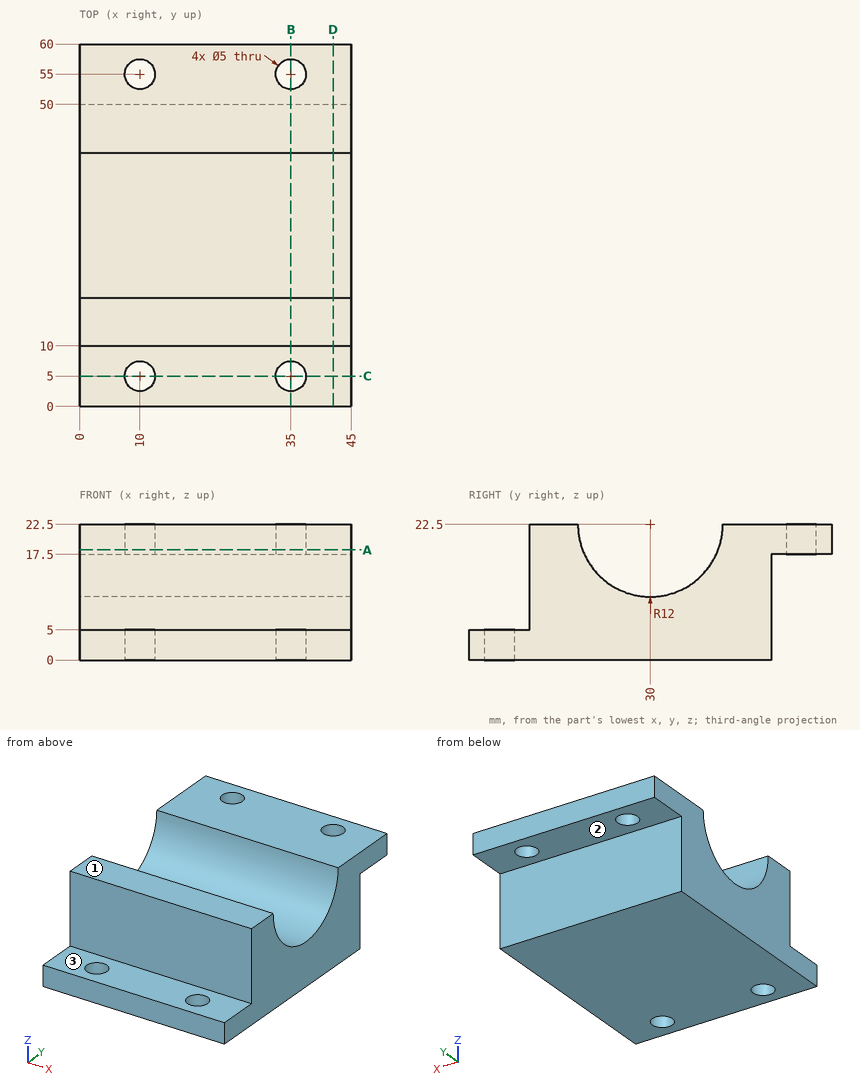
Can you work these out from the drawing? Everything is in mm from the part's minimum corner. A direction names the side the tool comes from. Give positions to 0.01 mm unless a question says otherwise; leave off trailing zeros. Loops run counter-clockwise (first coordinate to the right, second up) from the corner with the lowest first, then second, coordinate; pieces in that order, holes last. Notation, with made-up numbers: (49.5, -12) - (78.5, -12) arc R20 cw to (78.5, 12) - close; hole circle Ø6 at (70, 59.25). An arc over 180 degrees is marked (long way). Use one line per item in the form item = value.
1. I want a section at A-A (z = 18.25). Please give me the cut outline in (x, y).
Response values:
outline = (0, 10) - (45, 10) - (45, 18.78) - (0, 18.78) - close; (0, 41.22) - (45, 41.22) - (45, 60) - (0, 60) - close; hole circle Ø5 at (10, 55); hole circle Ø5 at (35, 55)
2. I'm going to push flat-ended pins straight in: pin 1 Ø4 at (x, z) = (34, 5.5) entering from +Y; pin 2 Ø8 at (x, y) = (35, 5) entering from -Z; pin 3 Ø8 at (x, y) = (31.5, 4) entering from +Z; pin 4 Ø8 at (x, y) = (10, 55) entering from -Z. Where does each tip first touch, or does it pass through?
Response values:
pin_1 = 50
pin_2 = 0
pin_3 = 5
pin_4 = 17.5
3. I want a section at D-D (x = 42). Please give me the cut outline in (y, z).
Response values:
outline = (0, 0) - (50, 0) - (50, 17.5) - (60, 17.5) - (60, 22.5) - (42, 22.5) arc R12 cw to (18, 22.5) - (10, 22.5) - (10, 5) - (0, 5) - close
4. On a 3-axis mill with a long thin cutter (end or side, diameter ignored), from which of +Z, -Z, +X, -X, +Y, -Y can I reach the whole of each face in a straight line? I mean the marked faces 1, 2 and 3. Say none if no direction works.
Response values:
face_1 = +Z, +X, -X, +Y, -Y
face_2 = -Z, +X, -X, +Y
face_3 = +Z, +X, -X, -Y
5. I need wall thicknesses on probe 1 along X at (y, z) = (55, 19.25); probe 2 along Z at (x, y) = (24.5, 57.5); probe 3 along Y at (x, z) = (31.5, 2.5). Which ranges of each line are inside material? Lowest first, please.
Response values:
probe_1 = 0 to 7.5, 12.5 to 32.5, 37.5 to 45
probe_2 = 17.5 to 22.5
probe_3 = 0 to 50
6. I want a section at C-C (y = 5). Please give me the cut outline in (x, z).
Response values:
outline = (0, 0) - (7.5, 0) - (7.5, 5) - (0, 5) - close; (12.5, 0) - (32.5, 0) - (32.5, 5) - (12.5, 5) - close; (37.5, 0) - (45, 0) - (45, 5) - (37.5, 5) - close
7. I want a section at B-B (x = 35). Please give me the cut outline in (y, z), and give its area (3 significant figures).
Response values:
outline = (0, 0) - (2.5, 0) - (2.5, 5) - (0, 5) - close; (7.5, 0) - (50, 0) - (50, 17.5) - (52.5, 17.5) - (52.5, 22.5) - (42, 22.5) arc R12 cw to (18, 22.5) - (10, 22.5) - (10, 5) - (7.5, 5) - close; (57.5, 17.5) - (60, 17.5) - (60, 22.5) - (57.5, 22.5) - close
area = 724 mm²
